from build123d import *

# Parameters (mm, degrees)
SKETCH_1_W          = 120
SKETCH_1_H          = 95
EXTRUDE_1_DEPTH     = 4
SKETCH_2_R          = 2.1
CUT_EXTRUDE_1_DEPTH = 10
SKETCH_3_R          = 2.05
CUT_EXTRUDE_2_DEPTH = 10
SKETCH_4_W          = 180
SKETCH_4_H          = 50.32629385
SKETCH_4_R          = 2.05
EXTRUDE_2_DEPTH     = 4
EXTRUDE_3_DEPTH     = 4
CUT_EXTRUDE_3_DEPTH = 10
FILLET_1_R          = 2
SKETCH_7_R          = 2.05
CUT_EXTRUDE_4_DEPTH = 10
FILLET_2_R          = 2
SKETCH_8_W          = 20
SKETCH_8_H          = 18
CUT_EXTRUDE_5_DEPTH = 10
SKETCH_9_W          = 38.5
SKETCH_9_H          = 26.173706147
CUT_EXTRUDE_6_DEPTH = 10
FILLET_3_R          = 3
SKETCH_10_R         = 2.05
CUT_EXTRUDE_7_DEPTH = 10
SKETCH_11_W         = 180
SKETCH_11_H         = 15
CUT_EXTRUDE_8_DEPTH = 10
FILLET_4_R          = 2


with BuildPart() as part:
    # 草图1 → 凸台-拉伸1 (new body)
    with BuildSketch(Plane.XY):
        Rectangle(SKETCH_1_W, SKETCH_1_H)
    extrude(amount=EXTRUDE_1_DEPTH)

    # 草图2 → 切除-拉伸1 (cut)
    with BuildSketch(Plane(origin=(0, 0, 0), x_dir=(-1, 0, 0), z_dir=(0, 0, -1))):
        with Locations((47.5, -40.326293853)):
            Circle(SKETCH_2_R)
        with Locations((47.5, -15.326293853)):
            Circle(SKETCH_2_R)
        with Locations((-47.5, -15.326293853)):
            Circle(SKETCH_2_R)
        with Locations((-47.5, -40.326293853)):
            Circle(SKETCH_2_R)
    extrude(amount=-CUT_EXTRUDE_1_DEPTH, mode=Mode.SUBTRACT)

    # 草图3 → 切除-拉伸2 (cut)
    with BuildSketch(Plane(origin=(0, 0, 0), x_dir=(-1, 0, 0), z_dir=(0, 0, -1))):
        with Locations((56, 33.17370615)):
            Circle(SKETCH_3_R)
        with Locations((-56, 33.17370615)):
            Circle(SKETCH_3_R)
        with Locations((-56, 5.17370615)):
            Circle(SKETCH_3_R)
        with Locations((56, 5.17370615)):
            Circle(SKETCH_3_R)
    extrude(amount=-CUT_EXTRUDE_2_DEPTH, mode=Mode.SUBTRACT)

    # 草图4 → 凸台-拉伸2 (add)
    with BuildSketch(Plane(origin=(0, 0, 0), x_dir=(-1, 0, 0), z_dir=(0, 0, -1))):
        with Locations((0, 22.336853075)):
            Rectangle(SKETCH_4_W, SKETCH_4_H)
        with Locations((56, 5.17370615)):
            Circle(SKETCH_4_R, mode=Mode.SUBTRACT)
        with Locations((56, 33.17370615)):
            Circle(SKETCH_4_R, mode=Mode.SUBTRACT)
        with Locations((-56, 5.17370615)):
            Circle(SKETCH_4_R, mode=Mode.SUBTRACT)
        with Locations((-56, 33.17370615)):
            Circle(SKETCH_4_R, mode=Mode.SUBTRACT)
    extrude(amount=-EXTRUDE_2_DEPTH)

    # 草图5 → 凸台-拉伸3 (add)
    with BuildSketch(Plane(origin=(0, 0, 0), x_dir=(-1, 0, 0), z_dir=(0, 0, -1))):
        Polygon((-90, -2.82629385), (-60, -47.5), (-60, -2.82629385), align=None)
        Polygon((60, -47.5), (60, -2.82629385), (90, -2.82629385), align=None)
    extrude(amount=-EXTRUDE_3_DEPTH)

    # 草图6 → 切除-拉伸3 (cut)
    with BuildSketch(Plane.XY.offset(4)):
        Polygon((-81.312928752, -5), (-53.5, -5), (-53.5, -46.416886874), align=None)
        Polygon((53.5, -46.416886874), (81.312928752, -5), (53.5, -5), align=None)
    extrude(amount=-CUT_EXTRUDE_3_DEPTH, mode=Mode.SUBTRACT)

    # 圆角1
    fillet_1_edges = [part.edges().sort_by_distance(p)[0] for p in [
        (-53.5, -46.416886874, 2),
        (-81.312928752, -5, 2),
        (-53.5, -5, 2),
        (53.5, -46.416886874, 2),
        (53.5, -5, 2),
        (81.312928752, -5, 2),
    ]]
    fillet(fillet_1_edges, radius=FILLET_1_R)

    # 草图7 → 切除-拉伸4 (cut)
    with BuildSketch(Plane.XY.offset(4)):
        with Locations((-84, 33.17370615)):
            Circle(SKETCH_7_R)
        with Locations((-84, 5.17370615)):
            Circle(SKETCH_7_R)
        with Locations(Location((84, 33.17370615, 0), (0, 0, 180))):
            Circle(SKETCH_7_R)
        with Locations(Location((84, 5.17370615, 0), (0, 0, 180))):
            Circle(SKETCH_7_R)
    extrude(amount=-CUT_EXTRUDE_4_DEPTH, mode=Mode.SUBTRACT)

    # 圆角2
    fillet_2_edges = [part.edges().sort_by_distance(p)[0] for p in [
        (-90, -2.82629385, 2),
        (90, 47.5, 2),
        (-90, 47.5, 2),
        (90, -2.82629385, 2),
        (60, -47.5, 2),
        (-60, -47.5, 2),
    ]]
    fillet(fillet_2_edges, radius=FILLET_2_R)

    # 草图8 → 切除-拉伸5 (cut)
    with BuildSketch(Plane.XY.offset(4)):
        with Locations((-70, 19.17370615)):
            Rectangle(SKETCH_8_W, SKETCH_8_H)
        Polygon((-48.5, 29.232984165), (-48.5, -6.059278018), (-7.576586563, 11.586853073), align=None)
        Polygon((-40.923413437, 32.5), (0, 14.853868908), (40.923413437, 32.5), align=None)
        Polygon((48.5, 29.232984165), (7.576586563, 11.586853073), (48.5, -6.059278018), align=None)
        Polygon((0, 8.319837238), (-40.923413437, -9.326293853), (40.923413437, -9.326293853), align=None)
        with Locations((70, 19.17370615)):
            Rectangle(SKETCH_8_W, SKETCH_8_H)
    extrude(amount=-CUT_EXTRUDE_5_DEPTH, mode=Mode.SUBTRACT)

    # 草图9 → 切除-拉伸6 (cut)
    with BuildSketch(Plane.XY.offset(4)):
        with Locations((-22.25, -28.413146927)):
            Rectangle(SKETCH_9_W, SKETCH_9_H)
        with Locations((22.25, -28.413146927)):
            Rectangle(SKETCH_9_W, SKETCH_9_H)
    extrude(amount=-CUT_EXTRUDE_6_DEPTH, mode=Mode.SUBTRACT)

    # 圆角3
    fillet_3_edges = [part.edges().sort_by_distance(p)[0] for p in [
        (-60, 10.17370615, 2),
        (-80, 10.17370615, 2),
        (-80, 28.17370615, 2),
        (-60, 28.17370615, 2),
        (7.576586563, 11.586853073, 2),
        (48.5, 29.232984165, 2),
        (48.5, -6.059278018, 2),
        (-40.923413437, -9.326293853, 2),
        (0, 8.319837238, 2),
        (40.923413437, -9.326293853, 2),
        (-48.5, -6.059278018, 2),
        (-48.5, 29.232984165, 2),
        (-7.576586563, 11.586853073, 2),
        (0, 14.853868908, 2),
        (-40.923413437, 32.5, 2),
        (40.923413437, 32.5, 2),
        (80, 10.17370615, 2),
        (60, 10.17370615, 2),
        (60, 28.17370615, 2),
        (80, 28.17370615, 2),
        (-3, -15.326293853, 2),
        (-3, -41.5, 2),
        (-41.5, -41.5, 2),
        (-41.5, -15.326293853, 2),
        (3, -15.326293853, 2),
        (41.5, -15.326293853, 2),
        (41.5, -41.5, 2),
        (3, -41.5, 2),
    ]]
    fillet(fillet_3_edges, radius=FILLET_3_R)

    # 草图10 → 切除-拉伸7 (cut)
    with BuildSketch(Plane.XY.offset(4)):
        with Locations((-66, 33.17370615)):
            Circle(SKETCH_10_R)
        with Locations((-66, 5.17370615)):
            Circle(SKETCH_10_R)
        with Locations(Location((66, 5.17370615, 0), (0, 0, 180))):
            Circle(SKETCH_10_R)
        with Locations(Location((66, 33.17370615, 0), (0, 0, 180))):
            Circle(SKETCH_10_R)
    extrude(amount=-CUT_EXTRUDE_7_DEPTH, mode=Mode.SUBTRACT)

    # 草图11 → 切除-拉伸8 (cut)
    with BuildSketch(Plane.XY.offset(4)):
        with Locations((0, 46.67370615)):
            Rectangle(SKETCH_11_W, SKETCH_11_H)
    extrude(amount=-CUT_EXTRUDE_8_DEPTH, mode=Mode.SUBTRACT)

    # 圆角4
    fillet_4_edges = [part.edges().sort_by_distance(p)[0] for p in [
        (-90, 39.17370615, 2),
        (90, 39.17370615, 2),
    ]]
    fillet(fillet_4_edges, radius=FILLET_4_R)


solid = part.part
Design review of the part built by this model. Coordinates are the model's own, in mm. A direction names the side the tool comes from. Round coordinates to 2 decimals unless told otherwise and drop trailing zeros. Write each loop counter-clockwise with the first axis right and the second up, starting at its lowest first coordinate (ties: lowest second). Pieces come first, ordered by that corner, then holes. Notation, with made-up numbers: (50, 35.5) - (84, 35.5) arc R25 ccw to (84, 72.5) - close; hole circle Ø3 at (69.5, -35). An arc over 180 degrees is marked (long way). Return JSON: item names as keys, results as strings. Group by question number.
Item 1: The part is to be moulded in two halves that separate along Y. For faces 3 (the face through (-1, -47.5, 2)), 4 (the face through (54.951, -41.774, 1.972)), 5 (the face through (47.114, 27.201, 1.972)), 6 (the face through (-90, 17, 2)), say which applies: pulls with the +Y half, pulls with the -Y half, needs draft (parallel to the pull), parting line crosses it, or undercut.
Item 2: We need section A-A on x = 19.5. Write out the cut boundary in (y, z), and give its area (3 significant figures).
Item 3: We need section D-D on z = 1.1. Give the number of separate pieces and of enclosed holes in the cut face, and give its area (3 significant figures).
Item 4: Insertion check: P1, Ø2, axis at x = -70.5, z = 1, coming from the -Y side; P2, Ø1.5, axis at x = -68.5, z = 2, coming from the -Y side; P3, Ø2, axis at y = -30, z = 2.5, coming from the +X side. Each pin has a flat end and moves straight along its axis. Give the tip position at first contact, or say it passes through.
Item 5: For probe 1 along X at (y, z) = (-24.5, 3.7); probe 2 along X at (y, z) = (-14.5, 1.1); probe 3 along Y at (x, z) = (-32, 0.5), list the stretches that pass through material, from the lowest coordinate up. Write a range as [from, to].
Item 6: We need section C-C on x = -84. Write out the cut boundary in (y, z), and give its area (3 significant figures).
Item 7: Machinability: for faces 1 (the face through (90, 17, 2)), 2 (the face through (-22, -41.5, 2)), which of the approach directions +Z, -Z, +X, -X, +Y, -Y give a long, thin tool a straight path to every point of the face, cutting with its end or side? Answer none if there is none.
Item 8: We need section B-B on y = 20. Write out the cut boundary in (x, z).
Model answer:
{
 "1": {"face 3": "pulls with the -Y half", "face 4": "undercut", "face 5": "undercut", "face 6": "needs draft"},
 "2": {"outline": "(-47.5, 0) - (-41.5, 0) - (-41.5, 4) - (-47.5, 4) - close; (-15.33, 0) - (-9.33, 0) - (-9.33, 4) - (-15.33, 4) - close; (-0.09, 0) - (6.45, 0) - (6.45, 4) - (-0.09, 4) - close; (16.73, 0) - (23.26, 0) - (23.26, 4) - (16.73, 4) - close; (32.5, 0) - (39.17, 0) - (39.17, 4) - (32.5, 4) - close", "area": "127 mm²"},
 "3": {"separate pieces": "1", "enclosed holes": "26", "area": "7,490 mm²"},
 "4": {"P1": "stops at y = -33.35", "P2": "stops at y = -35.96", "P3": "stops at x = 72.42"},
 "5": {"probe 1": "x = [-75.45, -68.22], [-53.5, -41.5], [-3, 3], [41.5, 53.5], [68.22, 75.45]", "probe 2": "x = [-82.16, -74.93], [-53.5, -49.43], [-45.57, 45.57], [49.43, 53.5], [74.93, 82.16]", "probe 3": "y = [-47.5, -41.5], [-15.33, 1.06], [22.12, 39.17]"},
 "6": {"outline": "(-11.76, 0) - (3.12, 0) - (3.12, 4) - (-11.76, 4) - close; (7.22, 0) - (31.12, 0) - (31.12, 4) - (7.22, 4) - close; (35.22, 0) - (39.17, 0) - (39.17, 4) - (35.22, 4) - close", "area": "171 mm²"},
 "7": {"face 1": "+Z, -Z, +X, +Y, -Y", "face 2": "+Z, -Z"},
 "8": {"outline": "(-90, 0) - (-80, 0) - (-80, 4) - (-90, 4) - close; (-60, 0) - (-48.5, 0) - (-48.5, 4) - (-60, 4) - close; (-27.09, 0) - (-11.93, 0) - (-11.93, 4) - (-27.09, 4) - close; (11.93, 0) - (27.09, 0) - (27.09, 4) - (11.93, 4) - close; (48.5, 0) - (60, 0) - (60, 4) - (48.5, 4) - close; (80, 0) - (90, 0) - (90, 4) - (80, 4) - close"}
}
